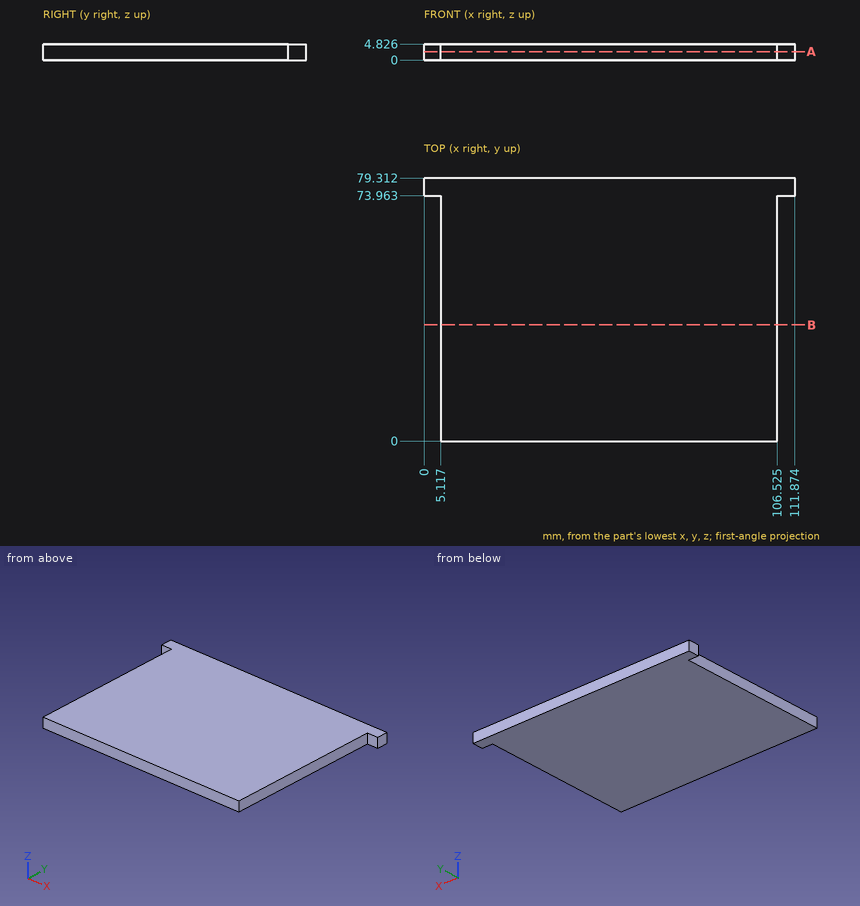
Can you work these out from the drawing? Everything is in mm from the part's minimum corner. Give positions to 0.01 mm unless a question says otherwise; leave off trailing zeros. Loops run counter-clockwise (first coordinate to the right, second up) from the corner with the lowest first, then second, coordinate; pieces in that order, holes last. Notation, with made-up numbers: (20, 20) - (31, 20) arc R17 cw to (31, 36) - close; hole circle Ø8 at (-28, 78.5). An arc over 180 degrees is marked (long way). Use one line per item in the form item = value.
1. I want a section at A-A (z = 2.5). Please give me the cut outline in (x, y) (1 decimal), and give its area (3 significant figures).
Response values:
outline = (0, 74) - (5.1, 74) - (5.1, 0) - (106.5, 0) - (106.5, 74) - (111.9, 74) - (111.9, 79.3) - (0, 79.3) - close
area = 8,100 mm²
2. I want a section at B-B (y = 35). Please give me the cut outline in (x, z) (1 decimal).
Response values:
outline = (5.1, 0) - (106.5, 0) - (106.5, 4.8) - (5.1, 4.8) - close
3. I need wall thicknesses on probe 1 along X at (y, z) = (22, 2.7) (1 decimal). Which ranges of the line are inside material? Lowest first, please.
Response values:
probe_1 = 5.1 to 106.5
4. I'm going to push flat-ended pins straight in: pin 1 Ø2.5 at (y, z) = (54, 2) entering from +X (1 decimal); pin 2 Ø1 at (y, z) = (14.5, 1.5) entering from -X; pin 3 Ø1.4 at (x, z) = (109, 1.5) entering from -Y. Where does each tip first touch, or does it pass through?
Response values:
pin_1 = 106.5
pin_2 = 5.12
pin_3 = 73.96
